Autodesk Inventor part; units mm, degrees
ref_plane "YZ Plane" through (0, 0, 0) normal (1, 0, 0) x (0, 1, 0)
ref_plane "XZ Plane" through (0, 0, 0) normal (0, 1, 0) x (-1, 0, 0)
ref_plane "XY Plane" through (0, 0, 0) normal (0, 0, 1) x (1, 0, 0)
sketch "Sketch1" plane through (0, 0, 0) normal (0, 1, 0) x (-1, 0, 0)
  line L0 (0, 0) -> (100, 0)
  line L1 (100, 0) -> (100, -1220)
  line L2 (100, -1220) -> (0, -1220)
  line L3 (0, -1220) -> (0, 0)
  dimension "d0" = 100
  dimension "d1" = 1220
extrude "Extrusion1" add sketch "Sketch1" along normal blind 10
ref_plane "Work Plane1" through (-50, 0, 0) normal (1, 0, 0) x (0, 0, -1)
sketch "Sketch2" plane through (-50, 0, 0) normal (1, 0, 0) x (0, 0, -1)
  line L0 (1220, 0) -> (0, 0)
  line L1 (1220, 0) -> (1220, 10)
  line L2 (0, 10) -> (1220, 10)
  line L3 (0, 0) -> (0, 10)
  line L4 (1220, 10) -> (1083.331, 10)
  line L5 (0, 10) -> (1220, 10)
  line L6 (1083.331, 10) -> (1183.331, 10) construction
  circle A0 centre (1083.331, 70) radius 2.5
  arc A1 (1087.331, 70) -> (1079.331, 70) centre (1083.331, 70) ccw
  line L7 (1087.331, 70) -> (1087.331, 10)
  line L8 (1087.331, 10) -> (1079.331, 10)
  line L9 (1079.331, 10) -> (1079.331, 70)
  dimension "d5" = 136.669
  dimension "d8" = 5
  dimension "d9" = 8
  dimension "d11" = 8
  dimension "d12" = 4
  dimension "d14" = 60
extrude "Extrusion2" add sketch "Sketch2" along normal mid plane 5 contours L2 L9 A1 L7
sketch "Sketch3" plane through (-50, 0, 0) normal (1, 0, 0) x (0, 0, -1)
  line L0 (1220, 0) -> (0, 0)
  line L1 (1220, 0) -> (1220, 10)
  line L2 (0, 10) -> (1220, 10)
  line L3 (0, 0) -> (0, 10)
  line L4 (1220, 10) -> (0, 10)
  line L5 (0, 10) -> (11.15, 10)
  circle A0 centre (11.15, 120) radius 2.5
  arc A1 (15.15, 120) -> (7.15, 120) centre (11.15, 120) ccw
  line L6 (15.15, 120) -> (15.15, 10)
  line L7 (15.15, 10) -> (7.15, 10)
  line L8 (7.15, 10) -> (7.15, 120)
  dimension "d18" = 11.15
  dimension "d21" = 5
  dimension "d22" = 8
  dimension "d24" = 8
  dimension "d31" = 110
extrude "Extrusion3" add sketch "Sketch3" along normal mid plane 10 contours L2 L8 A1 L6
sketch "Sketch4" plane through (-50, 0, 0) normal (1, 0, 0) x (0, 0, -1)
  arc A0 (15.15, 120) -> (7.15, 120) centre (11.15, 120) ccw
  circle A1 centre (11.15, 120) radius 2.5
  line L0 (7.15, 120) -> (7.15, 10)
  line L1 (15.15, 124) -> (7.15, 124)
  line L2 (7.15, 124) -> (7.15, 114)
  line L3 (7.15, 114) -> (15.15, 114)
  line L4 (15.15, 114) -> (15.15, 124)
  point P0 (0, 0)
  dimension "d27" = 10
  dimension "d30" = 4
extrude "Extrusion4" cut sketch "Sketch4" along normal mid plane 5
equation "\"d12\" = 0.5 * d11"
properties part number "Base"
Source: CAD feature listing. Evaluate the final solid. Frame: model axes, mm. Give positions to 0.01 mm unless a question says otherwise; leave off trailing zeros. Write each loop counter-clockwise with the first axis right and the second up, starting at its lowest first coordinate (ties: lowest second). Pieces come first, ordered by that corner, then holes.
1. First-contact query: pin 1 (1 mm diameter, centred on x = -27.5, z = -576.5, fed in from +Y); pin 2 (6.5 mm diameter, centred on y = 70, z = -12.5, fed in from -X); pin 3 (4.5 mm diameter, centred on y = 120, z = -11.15, fed in from -X); pin 4 (3 mm diameter, centred on x = -52, y = 78.5, fed in from -Z). Flat tips, straight axial feed; report the tip coordinate or a pass-through.
2. Section query A-A (z = -189.5). Return the cut outline in (x, y).
3. Material intervals for line 1 along Y through (x, z) = (-46.15, -11.15); line 2 along Y through (x, z) = (-17, -767), sorted ascending.
4. Section query B-B (x = -15.5). Return the cut outline in (y, z), then the cut area to 3 significant figures.
Output values:
1. pin 1: stops at y = 10
1. pin 2: stops at x = -55
1. pin 3: passes through
1. pin 4: stops at z = -15.15
2. outline: (-100, 0) - (0, 0) - (0, 10) - (-100, 10) - close
3. line 1: y = 0 to 117.5, 122.5 to 124
3. line 2: y = 0 to 10
4. outline: (0, -1220) - (10, -1220) - (10, 0) - (0, 0) - close
4. area: 12,200 mm2
